Build history of the part. All positions in model axes, mm. A direction names the side the tool comes from. Give positions to 0.01 mm unless a question says otherwise; leave off trailing zeros. Write each loop counter-clockwise with the first axis right and the second up, starting at its lowest first coordinate (ties: lowest second). Pieces come first, ordered by that corner, then holes. Notation, with made-up numbers: (86, -20.5) -> (96, -20.5) arc R18 cw to (96, 4.5) -> close; hole circle Ø1 at (39, 44.5). An arc over 180 degrees is marked (long way). Put each result on its own line as item: value.
Autodesk Inventor part; units mm, degrees
ref_plane "YZ Plane" through (0, 0, 0) normal (1, 0, 0) x (0, 1, 0)
ref_plane "XZ Plane" through (0, 0, 0) normal (0, 1, 0) x (-1, 0, 0)
ref_plane "XY Plane" through (0, 0, 0) normal (0, 0, 1) x (1, 0, 0)
sketch "Esquisse1" plane through (0, 0, 0) normal (0, 1, 0) x (-1, 0, 0)
  line L0 (55, -100) -> (-55, -100)
  line L1 (-55, -100) -> (-55, 100)
  line L2 (-55, 100) -> (55, 100)
  line L3 (55, 100) -> (55, -100)
  line L4 (55, -100) -> (-55, 100) construction
  line L5 (-55, -100) -> (55, 100) construction
  point P0 (0, 0)
  dimension "d0" = 110
  dimension "d1" = 200
extrude "Extrusion1" add sketch "Esquisse1" along normal blind 5
sketch "Esquisse6" plane through (-55, 0, 100) normal (0, 0, 1) x (1, 0, 0)
  line L0 (0, 0) -> (110, 0)
  line L1 (110, 0) -> (110, 5)
  line L2 (0, 5) -> (110, 5)
  line L3 (0, 0) -> (0, 5)
  point P0 (55, 0)
extrude "Extrusion2" add sketch "Esquisse6" along normal blind 40
sketch "Esquisse3" plane through (0, 0, 0) normal (0, -1, 0) x (1, 0, 0)
  line L0 (0, 0) -> (52.5, 0)
  line L1 (52.5, 0) -> (52.5, -97.5)
  line L2 (0, 28.6272) -> (0, -29.3855)
  line L3 (0, 0) -> (0, 137.5)
  line L4 (0, 137.5) -> (52.5, 137.5)
  point P0 (-52.5, -97.5)
  point P1 (-52.5, 137.5)
  dimension "d18" = 52.5
  dimension "d19" = 97.5
  dimension "d49" = 137.5
  dimension "d50" = 52.5
hole "Perçage2" at (52.5, 0, -97.5) at (-52.5, 0, -97.5) at (-52.5, 0, 137.5) at (52.5, 0, 137.5) direction (0, 1, 0) diameter 2.459 end through all
sketch "Esquisse5" plane through (0, 5, 0) normal (0, 1, 0) x (1, 0, 0)
  line L0 (0, 0) -> (-40, 0)
  line L1 (-40, 0) -> (-40, 65)
  line L2 (-40, 65) -> (40, 65)
  line L3 (40, 65) -> (40, -65)
  line L4 (40, -65) -> (-40, -65)
  line L5 (-40, -65) -> (-40, 0)
  dimension "d36" = 40
  dimension "d37" = 65
  dimension "d38" = 80
  dimension "d39" = 130
hole "Perçage4" at (-40, 5, -65) at (40, 5, -65) at (40, 5, 65) at (-40, 5, 65) direction (0, -1, 0) diameter 2.459 end through all
sketch "Esquisse4" plane through (0, 0, 0) normal (0, -1, 0) x (1, 0, 0)
  line L0 (0, 0) -> (0, 137.5)
  line L1 (0, 0) -> (87.5, 0)
  line L2 (0, 0) -> (0, -97.5)
  line L3 (55, -100) -> (-55, -100)
  point P0 (-87.5, 0)
  dimension "d27" = 137.5
  dimension "d28" = 87.5
  dimension "d51" = 97.5
hole "Perçage3" at (87.5, 0, 0) at (0, 0, 137.5) at (-87.5, 0, 0) at (0, 0, -97.5) direction (0, 1, 0) diameter 2.459 end through all
sketch "Esquisse7" plane through (0, 5, 0) normal (0, 1, 0) x (1, 0, 0)
  line L0 (55, 100) -> (-55, 100)
  line L1 (55, 100) -> (55, -140)
  line L2 (-55, 100) -> (55, 100)
  line L3 (55, 100) -> (55, 95)
  line L4 (55, 95) -> (-55, 95)
  line L5 (-55, 95) -> (-55, 100)
  point P0 (0, 0)
  dimension "d52" = 5
extrude "Extrusion3" cut sketch "Esquisse7" against normal blind 10
sketch "Esquisse8" plane through (0, 5, 0) normal (0, 1, 0) x (1, 0, 0)
  line L0 (-55, 95) -> (-55, -140)
  line L1 (-55, 95) -> (-55, 92.5)
  line L2 (-55, 92.5) -> (-52.5, 92.5)
  line L3 (55, 95) -> (55, -140)
  line L4 (55, 95) -> (52.5, 95)
  line L5 (-55, 95) -> (55, 95)
  line L6 (52.5, 95) -> (52.5, 92.5)
  point P0 (0, 0)
  dimension "d55" = 2.5
  dimension "d56" = 2.5
  dimension "d57" = 2.5
hole "Perçage5" at (-52.5, 5, -92.5) at (52.5, 5, -92.5) direction (0, -1, 0) diameter 2.459 end through all
sketch "Esquisse9" plane through (55, 5, -95) normal (0, 0, -1) x (-1, 0, 0)
  line L0 (0, -5) -> (0, 0)
  line L1 (0, 0) -> (5, 0)
  line L2 (0, 0) -> (110, 0)
  line L3 (5, 0) -> (5, -1)
  line L4 (5, -1) -> (25, -1)
  line L5 (25, -1) -> (25, -4)
  line L6 (25, -4) -> (5, -4)
  line L7 (5, -4) -> (5, -1)
  line L8 (110, 0) -> (105, 0)
  line L9 (105, 0) -> (105, -1)
  line L10 (105, -1) -> (85, -1)
  line L11 (85, -1) -> (85, -4)
  line L12 (85, -4) -> (105, -4)
  line L13 (105, -4) -> (105, -1)
  point P0 (55, -5)
  dimension "d65" = 5
  dimension "d66" = 1
  dimension "d67" = 20
  dimension "d68" = 3
  dimension "d69" = 5
  dimension "d70" = 20
extrude "Extrusion4" add sketch "Esquisse9" along normal blind 7
properties part number "chassis_bas"
1) Pin check, flat tips, straight feed: pin 1 (1.5 mm diameter, centred on y = 2, z = -97.5, fed in from +X); pin 2 (2.5 mm diameter, centred on y = 2.5, z = -100, fed in from -X); pin 3 (1.5 mm diameter, centred on x = -52.5, z = 137.5, fed in from -Y); pin 4 (5.5 mm diameter, centred on x = 39.5, z = -100, fed in from +Y). Stop position of each tip, or through.
Filled sheet:
pin 1: x = 50
pin 2: x = -50
pin 3: through
pin 4: y = 4
2) Slice it at A-A (y = 2.7). Give the number of separate pieces and of enclosed holes in the cut face, plus the area to 3 significant figures.
Filled sheet:
separate pieces: 1
enclosed holes: 9
area: 26,100 mm2
3) Tool access for faces 4 (the flat face through (-55, 2, 24)), 5 (the flat face through (-40, 1, -98)), 6 (the flat face through (40, 4, -98)): list every direction of +Z, -Z, +X, -X, +Y, -Y with a clear straight run to the whole face (end or side of a thin tool).
Filled sheet:
face 4: +Z, -Z, -X, +Y, -Y
face 5: -Z, +X, -X, -Y
face 6: -Z, +X, -X, +Y
4) Wall check: L1, parallel to Z at x = -40, y = 1.7; L2, parallel to Z at x = 52.5, y = 2.45; L3, parallel to X at y = 1.7, z = -92.5. Give the ranges that are in metal, low to high.
Filled sheet:
L1: -102 to -66.23, -63.77 to 63.77, 66.23 to 140
L2: -95 to -93.73, -91.27 to 136.27, 138.73 to 140
L3: -55 to -53.73, -51.27 to 51.27, 53.73 to 55
5) Slice it at B-B (x = 22.5). Write the cut outline in (y, z).
Filled sheet:
outline: (0, -95) -> (5, -95) -> (5, 140) -> (0, 140) -> close
6) Pull direction X, two halves, no side cores. Call faces 1 (the flat face through (1, 0, 24)), 2 (the flat face through (55, 2, 21)), 3 (the flat face through (1, 3, -95)): released by +X, released by -X, zero draft, split by the parting line, or undercut.
Filled sheet:
face 1: zero draft
face 2: released by +X
face 3: undercut
